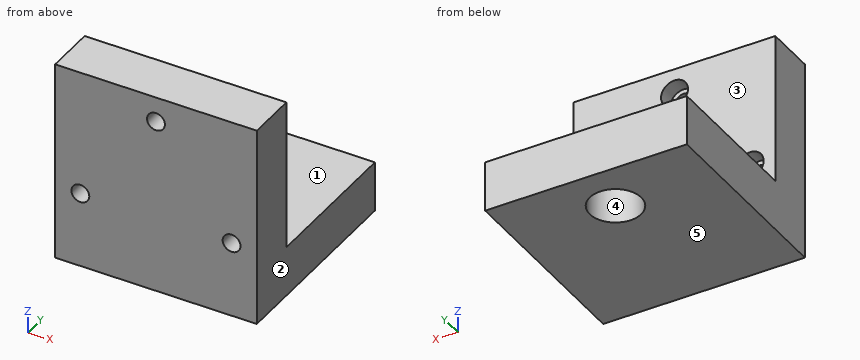
```python
from build123d import *

# Parameters (mm, degrees)
SKETCH1_W               = 25.4
SKETCH1_H               = 25.4
BOSS_EXTRUDE1_DEPTH     = 3.175
SKETCH2_W               = 25.4
SKETCH2_H               = 6.35
BOSS_EXTRUDE2_DEPTH     = 19.05
SKETCH4_R               = 1.127000032
CUT_EXTRUDE2_DEPTH      = 7.35
SKETCH9_R               = 1.700000029
CUT_EXTRUDE4_DEPTH      = 2.000000064
SKETCH3_R               = 3.2385
CUT_EXTRUDE1_DEPTH      = 20.05
CUT_EXTRUDE1_DEPTH_BACK = 7.35


with BuildPart() as part:
    # Sketch1 → Boss-Extrude1 (new body, symmetric)
    with BuildSketch(Plane.XY):
        with Locations((12.7, 12.7)):
            Rectangle(SKETCH1_W, SKETCH1_H)
    extrude(amount=BOSS_EXTRUDE1_DEPTH, both=True)

    # Sketch2 → Boss-Extrude2 (add)
    with BuildSketch(Plane.XY.offset(3.175)):
        with Locations((12.7, 3.175)):
            Rectangle(SKETCH2_W, SKETCH2_H)
    extrude(amount=BOSS_EXTRUDE2_DEPTH)

    # Sketch4 → Cut-Extrude2 (cut, through all)
    with BuildSketch(Plane(origin=(0, 6.35, 0), x_dir=(1, 0, 0), z_dir=(0, 1, 0))):
        with Locations((3.175, -6.35)):
            Circle(SKETCH4_R)
        with Locations((22.225, -6.35)):
            Circle(SKETCH4_R)
        with Locations((12.7, -19.05)):
            Circle(SKETCH4_R)
    extrude(amount=-CUT_EXTRUDE2_DEPTH, mode=Mode.SUBTRACT)

    # Sketch9 → Cut-Extrude4 (cut)
    with BuildSketch(Plane(origin=(0, 6.35, 0), x_dir=(1, 0, 0), z_dir=(0, 1, 0))):
        with Locations((3.175, -6.35)):
            Circle(SKETCH9_R)
        with Locations((22.225, -6.35)):
            Circle(SKETCH9_R)
        with Locations((12.7, -19.05)):
            Circle(SKETCH9_R)
    extrude(amount=-CUT_EXTRUDE4_DEPTH, mode=Mode.SUBTRACT)

    # Sketch3 → Cut-Extrude1 (cut, two sides)
    with BuildSketch(Plane.XY.offset(3.175)) as cut_extrude1_sk:
        with Locations((12.7, 19.05)):
            Circle(SKETCH3_R)
    extrude(amount=CUT_EXTRUDE1_DEPTH, mode=Mode.SUBTRACT)
    extrude(cut_extrude1_sk.sketch, amount=-CUT_EXTRUDE1_DEPTH_BACK, mode=Mode.SUBTRACT)


solid = part.part
```
Part model, mm, in its own coordinate system. Face numbers are marked on the shaded views. A direction names the side the tool comes from. Round coordinates to 2 decimals unless told otherwise and drop trailing zeros. Write each loop counter-clockwise with the first axis right and the second up, starting at its lowest first coordinate (ties: lowest second). Pieces come first, ordered by that corner, then holes. Notation, with made-up numbers: (8, 37) -> (38, 37) arc R11 ccw to (38, 57) -> close; hole circle Ø2 at (38.5, 53). An arc over 180 degrees is marked (long way). Return JSON: item names as keys, results as strings. Group by question number.
Q1. Probe L1, parallel to X at y = 4.9, z = 6.35 (3 decimals); L2, parallel to X at y = 3.15, z = 6.35; L3, parallel to Z at x = 12.7, y = 5.6 (3 decimals). List the from-to ranges inside material, lowest first. Write a range as [from, to].
Q2. Saw through at A-A on x = 12.7. State how many separate pieces and enclosed holes the cut face has, plus the area to 3 significant figures.
Q3. Pin check, flat tips, straight feed: pin 1 (2.5 mm diameter, centred on x = 13.5, z = 20, fed in from +Y); pin 2 (15 mm diameter, centred on x = 15, y = 17, fed in from +Z) (3 decimals). Stop position of each tip, or through.
Q4. Saw through at D-D on z = 19.05. Write the cut outline in (x, y).
Q5. Mould opens along Y. For the marked faces 3, 4 and 5 say: pulls with the +Y half, pulls with the -Y half, needs draft (parallel to the pull), parting line crosses it, or undercut.
Q6. Saw through at C-C on y = 19.05. Write the cut outline in (x, z) (1 decimal).
Q7. Which spindle directions (+Z, -Z, +X, -X, +Y, -Y) get a long thin tool onto all of the face, cutting with end or side? Do the marked faces 1 and 2. Say none if no direction does.
Q8. Saw through at B-B on z = 6.35. Write the cut outline in (x, y) (3 decimals), plus the area to 3 significant figures.
Answer:
{
 "1": {"L1": "[0, 1.475], [4.875, 20.525], [23.925, 25.4]", "L2": "[0, 2.05], [4.3, 21.1], [23.35, 25.4]", "L3": "[-3.175, 17.35], [20.75, 22.225]"},
 "2": {"separate pieces": "3", "enclosed holes": "0", "area": "225 mm2"},
 "3": {"pin 1": "y = 6.35", "pin 2": "z = 3.175"},
 "4": {"outline": "(0, 0) -> (11.57, 0) -> (11.57, 4.35) -> (11, 4.35) -> (11, 6.35) -> (0, 6.35) -> close; (13.83, 0) -> (25.4, 0) -> (25.4, 6.35) -> (14.4, 6.35) -> (14.4, 4.35) -> (13.83, 4.35) -> close"},
 "5": {"face 3": "pulls with the +Y half", "face 4": "undercut", "face 5": "needs draft"},
 "6": {"outline": "(0, -3.2) -> (9.5, -3.2) -> (9.5, 3.2) -> (0, 3.2) -> close; (15.9, -3.2) -> (25.4, -3.2) -> (25.4, 3.2) -> (15.9, 3.2) -> close"},
 "7": {"face 1": "+Z, +X, -X, +Y", "face 2": "+Z, -Z, +X, +Y, -Y"},
 "8": {"outline": "(0, 0) -> (2.048, 0) -> (2.048, 4.35) -> (1.475, 4.35) -> (1.475, 6.35) -> (0, 6.35) -> close; (4.302, 0) -> (21.098, 0) -> (21.098, 4.35) -> (20.525, 4.35) -> (20.525, 6.35) -> (4.875, 6.35) -> (4.875, 4.35) -> (4.302, 4.35) -> close; (23.352, 0) -> (25.4, 0) -> (25.4, 6.35) -> (23.925, 6.35) -> (23.925, 4.35) -> (23.352, 4.35) -> close", "area": "128 mm2"}
}
